The listing builds one solid part. Answer for the finished solid, in the listing's coordinates (mm). Face numbers are marked on the shaded views. A direction names the side the tool comes from. Coordinates: 2 decimals unless noted, no trailing zeros. Order: outer loops, then holes, each group sorted by start corner. A loop starts at its lowest first (then second) coordinate and runs counter-clockwise, first axis right, second up.
```python
from build123d import *

# Parameters (mm, degrees)
SKETCH064_R     = 5.25
PAD044_DEPTH    = 9
SKETCH065_R     = 2.75
POCKET016_DEPTH = 15.001
SKETCH066_R     = 6.5
POCKET017_DEPTH = 2
SKETCH067_R     = 9
PAD045_DEPTH    = 2
SKETCH068_W     = 9.725
SKETCH068_H     = 9.725
POCKET018_DEPTH = 4


with BuildPart() as part:
    # Sketch064 → Pad044 (new body, symmetric)
    with BuildSketch(Plane.XY):
        with BuildLine():
            Line((35, 15), (-35, 15))
            Line((-35, 15), (-35, 5))
            Line((-35, 5), (-9, 5))
            Line((-9, 5), (-9, 0))
            ThreePointArc((-9, 0), (0, -9), (9, 0))
            Line((9, 0), (9, 5))
            Line((9, 5), (35, 5))
            Line((35, 5), (35, 15))
        make_face()
        Circle(SKETCH064_R, mode=Mode.SUBTRACT)
    extrude(amount=PAD044_DEPTH, both=True)

    # Sketch065 → Pocket016 (cut, through all)
    with BuildSketch(Plane.XZ):
        with Locations((-25, 0)):
            Circle(SKETCH065_R)
        with Locations((25, 0)):
            Circle(SKETCH065_R)
    extrude(amount=-POCKET016_DEPTH, mode=Mode.SUBTRACT)

    # Sketch066 → Pocket017 (cut)
    with BuildSketch(Plane.XZ.offset(-15)):
        with Locations((-25, 0)):
            Circle(SKETCH066_R)
        with Locations((25, 0)):
            Circle(SKETCH066_R)
    extrude(amount=POCKET017_DEPTH, mode=Mode.SUBTRACT)

    # Sketch067 → Pad045 (join)
    with BuildSketch(Plane.XY.offset(-9)):
        Circle(SKETCH067_R)
    extrude(amount=PAD045_DEPTH)

    # Sketch068 → Pocket018 (cut)
    with BuildSketch(Plane.XZ.offset(-5)):
        with Locations((-25, 0)):
            Rectangle(SKETCH068_W, SKETCH068_H)
        with Locations((25, 0)):
            Rectangle(SKETCH068_W, SKETCH068_H)
    extrude(amount=-POCKET018_DEPTH, mode=Mode.SUBTRACT)


solid = part.part
```
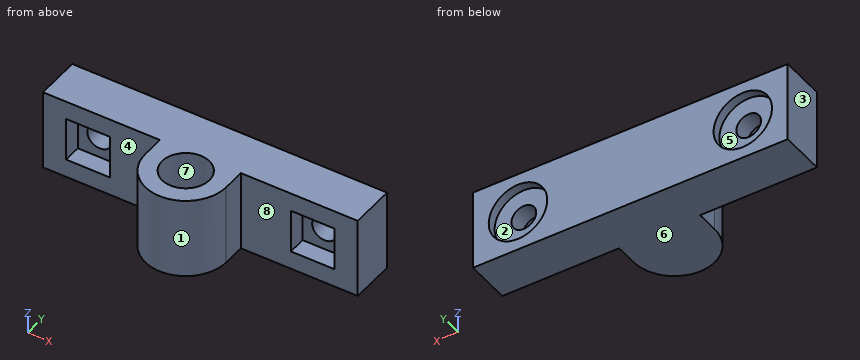
1) A cutting plane is placed at B-B, the plane z = 0. Count the separate pieces of the cut face and the enclosed holes in it, plus the area to 3 significant figures.
2) Each of these flat-tipped pins is pushed along its axis until it touches: P1, Ø3, axis at x = -26.5, z = -1.5, coming from the -Y side; P2, Ø1.5, axis at y = 2.5, z = 2.5, coming from the -X side; P3, Ø6.5, axis at x = 0, y = 0, coming from the +Z side. Where does it stop, or does it pass through?
3) The mould has two halves that part along X. Classify the marked faces 1, 2 and 3: released by +X, released by -X, zero draft, split by the parting line, or undercut.
4) A cutting plane is placed at A-A, the plane x = 25. Write down the section's boundary in (y, z), plus the area to 3 significant figures.
5) Straight lines are drawn through the part: probe 1 along Z at (x, y) = (25, 14.3); probe 2 along Z at (x, y) = (25, 9.8); probe 3 along X at (y, z) = (14.25, -5.5). For each, find the intervals that lie inside material, in ascending order.
6) A cutting plane is placed at D-D, the plane x = 0. Write down the section's boundary in (y, z).
7) A cutting plane is placed at C-C, the plane y = 7.75. Write down the section's boundary in (x, z).
8) For the marked faces 4, 5, 6, 7 and 8, determine the directions among +Z, -Z, +X, -X, +Y, -Y from which every point of the face is accessible in a straight line to the end or side of a thin tool.
Working result:
1. separate pieces: 3
1. enclosed holes: 1
1. area: 657 mm2
2. P1: stops at y = 9
2. P2: stops at x = -9
2. P3: stops at z = -7
3. face 1: split by the parting line
3. face 2: undercut
3. face 3: released by -X
4. outline: (5, -9) - (15, -9) - (15, -6.5) - (13, -6.5) - (13, -2.75) - (9, -2.75) - (9, -4.86) - (5, -4.86) - close; (5, 4.86) - (9, 4.86) - (9, 2.75) - (13, 2.75) - (13, 6.5) - (15, 6.5) - (15, 9) - (5, 9) - close
4. area: 93.1 mm2
5. probe 1: z = -9 to -6.5, 6.5 to 9
5. probe 2: z = -9 to -2.75, 2.75 to 9
5. probe 3: x = -35 to -28.46, -21.54 to 21.54, 28.46 to 35
6. outline: (-9, -9) - (15, -9) - (15, 9) - (5.25, 9) - (5.25, -7) - (-5.25, -7) - (-5.25, 9) - (-9, 9) - close
7. outline: (-35, -9) - (35, -9) - (35, 9) - (-35, 9) - close; hole (-29.86, -4.86) - (-20.14, -4.86) - (-20.14, 4.86) - (-29.86, 4.86) - close; hole (20.14, -4.86) - (29.86, -4.86) - (29.86, 4.86) - (20.14, 4.86) - close
8. face 4: +Z, -Z, -X, -Y
8. face 5: +Y
8. face 6: -Z, +X, -X, +Y, -Y
8. face 7: +Z
8. face 8: +Z, -Z, +X, -Y
